```python
from build123d import *

# Parameters (mm, degrees)
SKETCH1_R           = 7
BOSS_EXTRUDE1_DEPTH = 32.7
SKETCH4_W           = 23
SKETCH4_H           = 20
SKETCH4_R           = 3.5
BOSS_EXTRUDE2_DEPTH = 3.3
FILLET1_R           = 3
SKETCH5_R           = 1
CUT_EXTRUDE3_DEPTH  = 5
SKETCH2_R           = 4.6
CUT_EXTRUDE4_DEPTH  = 5
SKETCH6_R           = 2.75
CUT_EXTRUDE5_DEPTH  = 36
FILLET2_R           = 1
CHAMFER1_SIZE       = 0.8


with BuildPart() as part:
    # Sketch1 → Boss-Extrude1 (new body)
    with BuildSketch(Plane(origin=(0, 0, 0), x_dir=(1, 0, 0), z_dir=(0, 1, 0))):
        with Locations(Location((0, 0, 0), (0, 0, 270))):
            Circle(SKETCH1_R)
    extrude(amount=BOSS_EXTRUDE1_DEPTH)

    # Sketch4 → Boss-Extrude2 (add)
    with BuildSketch(Plane(origin=(0, 32.7, 0), x_dir=(1, 0, 0), z_dir=(0, 1, 0))):
        with Locations((1.5, 0)):
            Rectangle(SKETCH4_W, SKETCH4_H)
        Circle(SKETCH4_R, mode=Mode.SUBTRACT)
    extrude(amount=-BOSS_EXTRUDE2_DEPTH)

    # Fillet1
    fillet1_edges = [part.edges().sort_by_distance(p)[0] for p in [
        (-10, 31.05, 10),
        (-10, 31.05, -10),
        (13, 31.05, -10),
        (13, 31.05, 10),
    ]]
    fillet(fillet1_edges, radius=FILLET1_R)

    # Sketch5 → Cut-Extrude3 (cut)
    with BuildSketch(Plane(origin=(0, 32.7, 0), x_dir=(1, 0, 0), z_dir=(0, 1, 0))):
        with Locations(Location((-7, 7, 0), (0, 0, 270))):
            Circle(SKETCH5_R)
        with Locations(Location((10, 7, 0), (0, 0, 270))):
            Circle(SKETCH5_R)
        with Locations(Location((10, -7, 0), (0, 0, 270))):
            Circle(SKETCH5_R)
        with Locations(Location((-7, -7, 0), (0, 0, 270))):
            Circle(SKETCH5_R)
    extrude(amount=-CUT_EXTRUDE3_DEPTH, mode=Mode.SUBTRACT)

    # Sketch2 → Cut-Extrude4 (cut)
    with BuildSketch(Plane.XZ):
        with Locations(Location((0, 0, 0), (0, 0, 270))):
            Circle(SKETCH2_R)
    extrude(amount=-CUT_EXTRUDE4_DEPTH, mode=Mode.SUBTRACT)

    # Sketch6 → Cut-Extrude5 (cut)
    with BuildSketch(Plane.XZ.offset(-5)):
        with Locations(Location((0, 0, 0), (0, 0, 270))):
            Circle(SKETCH6_R)
    extrude(amount=-CUT_EXTRUDE5_DEPTH, mode=Mode.SUBTRACT)

    # Fillet2
    fillet2_edges = [part.edges().sort_by_distance(p)[0] for p in [
        (0, 29.4, -7),
    ]]
    fillet(fillet2_edges, radius=FILLET2_R)

    # Chamfer1
    chamfer1_edges = [part.edges().sort_by_distance(p)[0] for p in [
        (-7, 32.7, 6),
        (10, 32.7, 6),
        (10, 32.7, -8),
        (-7, 32.7, -8),
    ]]
    chamfer(chamfer1_edges, length=CHAMFER1_SIZE)


solid = part.part
```
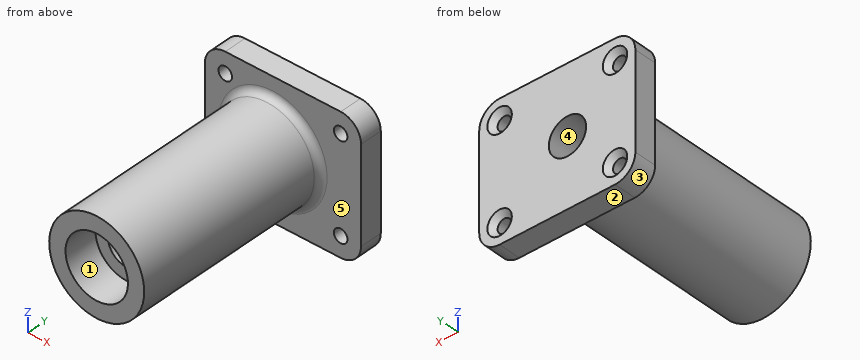
The listing builds one solid part. Answer for the finished solid, in the listing's coordinates (mm). Face numbers are marked on the shaded views. A direction names the side the tool comes from. Round coordinates to 2 decimals unless told otherwise and drop trailing zeros. Loops run counter-clockwise (first coordinate to the right, second up) from the corner with the lowest first, then second, coordinate; pieces in that order, holes last. Notation, with made-up numbers: (58, -16.5) -> (110, -16.5) arc R27 ccw to (110, 20.5) -> close; hole circle Ø1 at (84, 4.25). An arc over 180 degrees is marked (long way). Use one line per item in the form item = value.
1. Find the intervals of material crossed by probe 1 along X at (y, z) = (30.3, 7); probe 2 along X at (y, z) = (1.55, 0); probe 3 along Y at (x, z) = (7.25, -7.5), in increasing order. Write a range as [from, to].
Answer key:
probe_1 = [-10, -8], [-6, 9], [11, 13]
probe_2 = [-7, -4.6], [4.6, 7]
probe_3 = [29.4, 32.7]
2. The part is cut by section C-C on y = 13.5. Determine the outline of the cut face in (x, z).
Answer key:
outline = circle Ø14 at (0, 0); hole circle Ø5.5 at (0, 0)
3. For a pull along Z with two mould halves and no side action, classify the marked faces 3, 4 and 5 as released by +Z, released by -Z, zero draft, split by the parting line, or undercut.
Answer key:
face_3 = released by -Z
face_4 = undercut
face_5 = zero draft
4. Flat-ended cylindrical pins translate along their axes: pin 1 Ø4 at (x, y) = (-5.5, 5.5) entering from +Z; pin 2 Ø2.5 at (x, z) = (10, 7) entering from +Y; pin 3 Ø4.5 at (x, z) = (-1.5, -1) entering from -Y; pin 4 Ø4 at (x, y) = (9.5, 4) entering from +Z. Find the tip coordinate at first contact, or state that the pin passes through.
Answer key:
pin_1 = 6.06
pin_2 = 32.15
pin_3 = 5
pin_4 = through
5. The part is cut by section A-A on z = 0. Determine the outline of the cut face in (x, y).
Answer key:
outline = (-10, 29.4) -> (-8, 29.4) arc R1 cw to (-7, 28.4) -> (-7, 0) -> (-4.6, 0) -> (-4.6, 5) -> (-2.75, 5) -> (-2.75, 32.7) -> (-10, 32.7) -> close; (2.75, 5) -> (4.6, 5) -> (4.6, 0) -> (7, 0) -> (7, 28.4) arc R1 cw to (8, 29.4) -> (13, 29.4) -> (13, 32.7) -> (2.75, 32.7) -> close
6. A tool of negligible diameter and unlimited length cuts with its end or side. For the marked faces 1 and 2, from which of +Z, -Z, +X, -X, +Y, -Y can it reach the whole face along a straight path? Write none if from no direction.
Answer key:
face_1 = -Y
face_2 = -Z, +X, -X, +Y, -Y
7. The part is cut by section B-B on y = 30. Determine the outline of the cut face in (x, z).
Answer key:
outline = (-10, -7) arc R3 ccw to (-7, -10) -> (10, -10) arc R3 ccw to (13, -7) -> (13, 7) arc R3 ccw to (10, 10) -> (-7, 10) arc R3 ccw to (-10, 7) -> close; hole circle Ø2 at (-7, -7); hole circle Ø2 at (-7, 7); hole circle Ø5.5 at (0, 0); hole circle Ø2 at (10, -7); hole circle Ø2 at (10, 7)
